Design review of the part built by this model. Coordinates are the model's own, in mm. Face numbers are marked on the shaded views. A direction names the side the tool comes from. Round coordinates to 2 decimals unless told otherwise and drop trailing zeros. Loops run counter-clockwise (first coordinate to the right, second up) from the corner with the lowest first, then second, coordinate; pieces in that order, holes last. Notation, with made-up numbers: (24.25, -30) -> (62.25, -30) arc R15 ccw to (62.25, -21) -> close; hole circle Ø4 at (62, 49.25). An arc over 180 degrees is marked (long way). Use a Markdown table: item, result. Add a question column.
from build123d import *

# Parameters (mm, degrees)
F1_DEPTH = 40
F2_R     = 4.99999


# Not quite as in the source:
# - a fillet or chamfer is up to 0.001 mm smaller than in the source, because OpenCascade refuses the exact size


with BuildPart() as f1:
    # F0 (on Top) → F1 (new body)
    with BuildSketch(Plane.XY):
        Polygon((-27.5, -14.525), (27.5, -14.525), (27.5, 14.525), (27.5, 22.525), (22.5, 31.1852540378), (22.5, 22.525), (22.5, 14.525), (-27.5, 14.525), (-27.5, 9.525), (22.5, 9.525), (22.5, -9.525), (-27.5, -9.525), align=None)
    extrude(amount=F1_DEPTH)

    # F2 (radius 5 in the source; OpenCascade refuses exactly that, so slightly less here)
    f2_edges = [f1.edges().sort_by_distance(p)[0] for p in [
        (-27.5, 14.525, 20),
        (-27.5, -14.525, 20),
        (27.5, -14.525, 20),
        (27.5, 22.525, 20),
        (22.5, 14.525, 20),
    ]]
    fillet(f2_edges, radius=F2_R)


solid = f1.part
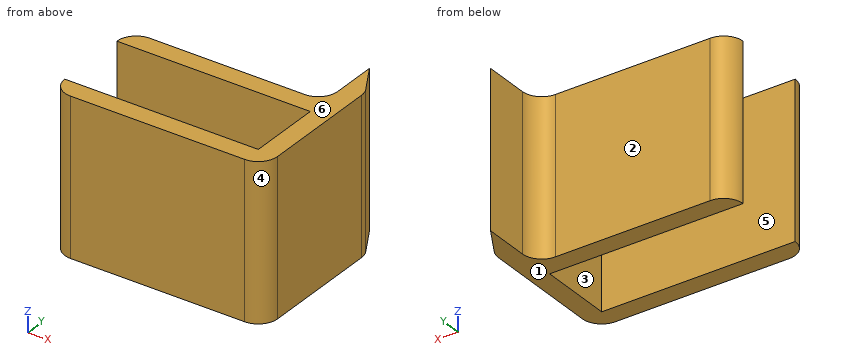
1. Mouldability with a two-part tool opening along Y and no side actions: class the marked faces 4, 5 and 6 as +Y half, -Y half, draft (parallel to the pull), parting line (faces both ways), or undercut.
2. Consider section A-A on x = 4. State the section outline as (y, z) points (3 decimals), plus the area to 3 significant figures.
3. Consider section C-C on y = 4.5. State the section outline as (x, z) points, plus the area to 3 significant figures.
4. Insertion check: P1, Ø15, axis at y = 1, z = 24, coming from the -X side; P2, Ø8, axis at x = 16.5, z = 12.5, coming from the +Y side (3 decimals); P3, Ø6, axis at x = 13, z = 15, coming from the +Y side (3 decimals). Each pin has a flat end and moves straight along its axis. Give the tip position at first contact, or say it passes through.
5. Consider section D-D on x = 19.5. State the section outline as (y, z) points (3 decimals).
6. To check wall thickness, follow probe 1 along Y at (x, z) = (12, 12) (3 decimals); probe 2 along X at (y, z) = (-5.5, 4.5); probe 3 along Y at (x, z) = (19.5, 6) (3 decimals). State the ranges of each line that lie inside material, in increasing order. Write a range as from..to.
7. For the marked faces 1, 2 and 3, list the 3-axis set-ups (+Z, -Z, +X, -X, +Y, -Y) from which the entire face can be reached by the end or side of a thin tool; tool diameter is ignored.
Verdict:
| question | item | result |
|---|---|---|
| 1 | face 4 | -Y half |
| 1 | face 5 | undercut |
| 1 | face 6 | draft |
| 2 | outline | (-14.525, 0) -> (-9.525, 0) -> (-9.525, 40) -> (-14.525, 40) -> close; (9.525, 0) -> (14.525, 0) -> (14.525, 40) -> (9.525, 40) -> close |
| 2 | area | 400 mm² |
| 3 | outline | (22.5, 0) -> (27.5, 0) -> (27.5, 40) -> (22.5, 40) -> close |
| 3 | area | 200 mm² |
| 4 | P1 | stops at x = 22.5 |
| 4 | P2 | stops at y = 15.525 |
| 4 | P3 | stops at y = 14.525 |
| 5 | outline | (-14.525, 0) -> (-9.525, 0) -> (-9.525, 40) -> (-14.525, 40) -> close; (9.525, 0) -> (14.942, 0) -> (14.942, 40) -> (9.525, 40) -> close |
| 6 | probe 1 | y = -14.525..-9.525, 9.525..14.525 |
| 6 | probe 2 | x = 22.5..27.5 |
| 6 | probe 3 | y = -14.525..-9.525, 9.525..14.942 |
| 7 | face 1 | -Z, +X, -X, +Y, -Y |
| 7 | face 2 | +Z, -Z, -X, +Y |
| 7 | face 3 | +Z, -Z, -X |
